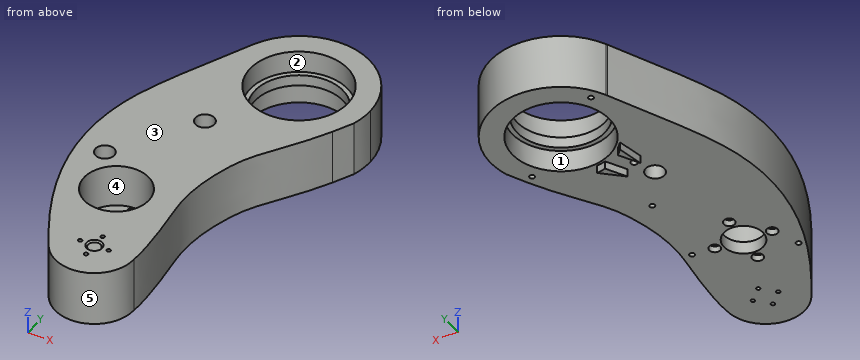
from build123d import *

# Parameters (mm, degrees)
SKIZZE1_R                        = 9
SKIZZE1_R_2                      = 28
AUFSATZ_LINEAR_AUSTRAGEN1_DEPTH  = 35
SKIZZE2_R                        = 4
SCHNITT_LINEAR_AUSTRAGEN1_DEPTH  = 1
FASE1_SIZE                       = 1
SKIZZE4_R                        = 1.25
SCHNITT_LINEAR_AUSTRAGEN2_DEPTH  = 15
SKIZZE5_R                        = 1.25
SCHNITT_LINEAR_AUSTRAGEN3_DEPTH  = 15
SKIZZE6_R                        = 12.5
SCHNITT_LINEAR_AUSTRAGEN4_DEPTH  = 35
SKIZZE7_R                        = 20.5
SCHNITT_LINEAR_AUSTRAGEN5_DEPTH  = 27
SKIZZE8_R                        = 2
SCHNITT_LINEAR_AUSTRAGEN6_DEPTH  = 15
SKIZZE9_R                        = 3.5
SCHNITT_LINEAR_AUSTRAGEN7_DEPTH  = 4
SKIZZE10_R                       = 31
SCHNITT_LINEAR_AUSTRAGEN8_DEPTH  = 14
SKIZZE11_R                       = 1.65
SCHNITT_LINEAR_AUSTRAGEN10_DEPTH = 15
SKIZZE12_R                       = 2.1
SCHNITT_LINEAR_AUSTRAGEN11_DEPTH = 15
BOSS_EXTRUDE1_DEPTH              = 5
SKETCH2_R                        = 6
CUT_EXTRUDE1_DEPTH               = 35
CUT_EXTRUDE2_START               = 8
SKETCH3_R                        = 6
CUT_EXTRUDE2_DEPTH               = 8
CUT_EXTRUDE3_START               = -10
SKETCH4_R                        = 6
CUT_EXTRUDE3_DEPTH               = 10
SKIZZE13_R                       = 1.65
SCHNITT_LINEAR_AUSTRAGEN12_DEPTH = 15


with BuildPart() as part:
    # Skizze1 → Aufsatz-Linear austragen1 (new body)
    # profile 1 of 4: a face of its own
    with BuildSketch(Plane.XY):
        with BuildLine():
            add(Edge.make_bspline(
                [(-21.90615173, -12.046597711), (-21.575742026, -12.598438537), (-21.248020936, -13.143822016), (-20.923299769, -13.682672501)],
                knots=[0.9859462, 0.9859462, 0.9859462, 0.9859462, 1, 1, 1, 1], degree=3))
            ThreePointArc((-20.923299769, -13.682672501), (7.138539969, -23.959157897), (25, 0))
            ThreePointArc((25, 0), (-6.218770247, 24.21418792), (-21.90615173, -12.046597711))
        make_face()
        Circle(SKIZZE1_R, mode=Mode.SUBTRACT)
    # profile 2 of 4: a face of its own
    with BuildSketch(Plane.XY):
        Circle(SKIZZE1_R)
    # profile 3 of 4: a face of its own
    with BuildSketch(Plane.XY):
        with BuildLine():
            ThreePointArc((-21.90615173, -12.046597711), (-6.218770247, 24.21418792), (25, 0))
            add(Edge.make_bspline(
                [(61.420827626, 153.570408345), (47.913273557, 128.743473036), (35.386108163, 117.222864261), (25.006140509, 88.46764169), (20.036125276, 66.269671918), (25.663716119, 21.50596296), (25.709290114, 4.90404347), (25, 0)],
                knots=[0.045529733, 0.045529733, 0.045529733, 0.045529733, 0.347734035, 0.409134766, 0.591243699, 0.652606584, 1, 1, 1, 1], degree=3))
            ThreePointArc((61.420827626, 153.570408345), (1.91364242, 141.373324067), (-15.526505959, 199.560222769))
            add(Edge.make_bspline(
                [(-15.526505959, 199.560222769), (-37.33502728, 155.24670183), (-72.898560815, 80.515220187), (-39.634443124, 17.562686966), (-21.90615173, -12.046597711)],
                knots=[0.001075204, 0.001075204, 0.001075204, 0.001075204, 0.231882812, 0.9859462, 0.9859462, 0.9859462, 0.9859462], degree=3))
        make_face()
    # profile 4 of 4: a face of its own
    with BuildSketch(Plane.XY):
        with BuildLine():
            ThreePointArc((-15.526505959, 199.560222769), (1.91364242, 141.373324067), (61.420827626, 153.570408345))
            add(Edge.make_bspline(
                [(67.734061127, 165.90035392), (65.561159832, 161.397385892), (63.455859297, 157.310804229), (61.420827626, 153.570408345)],
                knots=[0, 0, 0, 0, 0.045529733, 0.045529733, 0.045529733, 0.045529733], degree=3))
            ThreePointArc((67.734061127, 165.90035392), (69.429904067, 172.859718168), (70, 180))
            ThreePointArc((70, 180), (35.369713301, 223.788914648), (-15.220846491, 200.181266251))
            add(Edge.make_bspline(
                [(-15.220846491, 200.181266251), (-15.323026036, 199.973668406), (-15.424912199, 199.766654794), (-15.526505959, 199.560222769)],
                knots=[0, 0, 0, 0, 0.001075204, 0.001075204, 0.001075204, 0.001075204], degree=3))
        make_face()
        with Locations((25, 180)):
            Circle(SKIZZE1_R_2, mode=Mode.SUBTRACT)
    extrude(amount=AUFSATZ_LINEAR_AUSTRAGEN1_DEPTH)

    # Skizze2 → Schnitt-Linear austragen1 (cut)
    with BuildSketch(Plane.XY.offset(35)):
        Circle(SKIZZE2_R)
    extrude(amount=-SCHNITT_LINEAR_AUSTRAGEN1_DEPTH, mode=Mode.SUBTRACT)

    # Fase1
    fase1_edges = [part.edges().sort_by_distance(p)[0] for p in [
        (-4, 0, 35),
    ]]
    chamfer(fase1_edges, length=FASE1_SIZE - 0.0001)  # a hair under: the kernel refuses the full size

    # Skizze4 → Schnitt-Linear austragen2 (cut)
    with BuildSketch(Plane.XY.offset(35)):
        with Locations((0, 9)):
            Circle(SKIZZE4_R)
        with Locations((9, 0)):
            Circle(SKIZZE4_R)
        with Locations((0, -9)):
            Circle(SKIZZE4_R)
        with Locations((-9, 0)):
            Circle(SKIZZE4_R)
    extrude(amount=-SCHNITT_LINEAR_AUSTRAGEN2_DEPTH, mode=Mode.SUBTRACT)

    # Skizze5 → Schnitt-Linear austragen3 (cut)
    with BuildSketch(Plane(origin=(0, 0, 0), x_dir=(-1, 0, 0), z_dir=(0, 0, -1))):
        with Locations((8, 0)):
            Circle(SKIZZE5_R)
        with Locations((0, -8)):
            Circle(SKIZZE5_R)
        with Locations((-8, 0)):
            Circle(SKIZZE5_R)
        with Locations((0, 8)):
            Circle(SKIZZE5_R)
    extrude(amount=-SCHNITT_LINEAR_AUSTRAGEN3_DEPTH, mode=Mode.SUBTRACT)

    # Skizze6 → Schnitt-Linear austragen4 (cut)
    with BuildSketch(Plane.XY.offset(35)):
        with Locations((-15, 50)):
            Circle(SKIZZE6_R)
    extrude(amount=-SCHNITT_LINEAR_AUSTRAGEN4_DEPTH, mode=Mode.SUBTRACT)

    # Skizze7 → Schnitt-Linear austragen5 (cut)
    with BuildSketch(Plane.XY.offset(35)):
        with Locations((-15, 50)):
            Circle(SKIZZE7_R)
    extrude(amount=-SCHNITT_LINEAR_AUSTRAGEN5_DEPTH, mode=Mode.SUBTRACT)

    # Skizze8 → Schnitt-Linear austragen6 (cut)
    with BuildSketch(Plane.XY.offset(8)):
        with Locations((2.46462713, 51.112114754)):
            Circle(SKIZZE8_R)
        with Locations((-16.112114754, 67.46462713)):
            Circle(SKIZZE8_R)
        with Locations((-13.887885246, 32.53537287)):
            Circle(SKIZZE8_R)
        with Locations((-32.46462713, 48.887885246)):
            Circle(SKIZZE8_R)
    extrude(amount=-SCHNITT_LINEAR_AUSTRAGEN6_DEPTH, mode=Mode.SUBTRACT)

    # Skizze9 → Schnitt-Linear austragen7 (cut)
    with BuildSketch(Plane(origin=(0, 0, 0), x_dir=(-1, 0, 0), z_dir=(0, 0, -1))):
        with Locations((13.887885246, 32.53537287)):
            Circle(SKIZZE9_R)
        with Locations((-2.46462713, 51.112114754)):
            Circle(SKIZZE9_R)
        with Locations((16.112114754, 67.46462713)):
            Circle(SKIZZE9_R)
        with Locations((32.46462713, 48.887885246)):
            Circle(SKIZZE9_R)
    extrude(amount=-SCHNITT_LINEAR_AUSTRAGEN7_DEPTH, mode=Mode.SUBTRACT)

    # Skizze10 → Schnitt-Linear austragen8 (cut)
    with BuildSketch(Plane.XY.offset(35)):
        with Locations((25, 180)):
            Circle(SKIZZE10_R)
    schnitt_linear_austragen8 = extrude(amount=-SCHNITT_LINEAR_AUSTRAGEN8_DEPTH, mode=Mode.SUBTRACT)

    # Spiegeln1: Schnitt-Linear austragen8 across plane
    add(schnitt_linear_austragen8.mirror(Plane.XY.offset(17.5)), mode=Mode.SUBTRACT)

    # Skizze11 → Schnitt-Linear austragen10 (cut)
    with BuildSketch(Plane.XY):
        with Locations((12.868875195, 101.386680064)):
            Circle(SKIZZE11_R)
    extrude(amount=SCHNITT_LINEAR_AUSTRAGEN10_DEPTH, mode=Mode.SUBTRACT)

    # Skizze12 → Schnitt-Linear austragen11 (cut)
    with BuildSketch(Plane(origin=(0, 0, 0), x_dir=(-1, 0, 0), z_dir=(0, 0, -1))):
        with Locations((-2, 140)):
            Circle(SKIZZE12_R)
    extrude(amount=-SCHNITT_LINEAR_AUSTRAGEN11_DEPTH, mode=Mode.SUBTRACT)

    # Sketch1 → Boss-Extrude1 (add)
    with BuildSketch(Plane(origin=(0, 0, 0), x_dir=(-1, 0, 0), z_dir=(0, 0, -1))):
        with BuildLine():
            Line((-8.068344121, 136.51070213), (-15.214181441, 148.938245296))
            ThreePointArc((-15.214181441, 148.938245296), (-18.014496555, 148.191234041), (-20.870136061, 147.696144595))
            Line((-20.870136061, 147.696144595), (-8.068344121, 136.51070213))
        make_face()
        with BuildLine():
            ThreePointArc((0.443638721, 159.672282499), (-1.242605981, 157.724877562), (-3.077493199, 155.916841035))
            Line((-3.077493199, 155.916841035), (4.052249922, 143.517287782))
            Line((4.052249922, 143.517287782), (0.443638721, 159.672282499))
        make_face()
    extrude(amount=BOSS_EXTRUDE1_DEPTH)

    # Sketch2 → Cut-Extrude1 (cut)
    with BuildSketch(Plane(origin=(0, 0, 0), x_dir=(-1, 0, 0), z_dir=(0, 0, -1))):
        with Locations((3.710410677, 126.992836719)):
            Circle(SKETCH2_R)
    extrude(amount=-CUT_EXTRUDE1_DEPTH, mode=Mode.SUBTRACT)

    # Sketch3 → Cut-Extrude2 (cut)
    with BuildSketch(Plane(origin=(0, 0, 17.5), x_dir=(-1, 0, 0), z_dir=(0, 0, -1)).offset(CUT_EXTRUDE2_START)):
        with BuildLine():
            ThreePointArc((32.070234604, 72.232513918), (33.839840892, 80.53121825), (42.138545224, 78.761611961))
            Line((42.138545224, 78.761611961), (8.744565987, 130.257385741))
            ThreePointArc((8.744565987, 130.257385741), (9.463884926, 128.69505118), (9.710410677, 126.992836719))
            ThreePointArc((9.710410677, 126.992836719), (5.412625137, 121.23936247), (-1.323744633, 123.728287698))
            Line((-1.323744633, 123.728287698), (32.070234604, 72.232513918))
        make_face()
        with Locations((37.104389914, 75.497062939)):
            Circle(SKETCH3_R)
    extrude(amount=-CUT_EXTRUDE2_DEPTH, mode=Mode.SUBTRACT)

    # Sketch4 → Cut-Extrude3 (cut)
    with BuildSketch(Plane.XY.offset(35).offset(CUT_EXTRUDE3_START)):
        with Locations((-37.104389914, 75.497062939)):
            Circle(SKETCH4_R)
    extrude(amount=CUT_EXTRUDE3_DEPTH, mode=Mode.SUBTRACT)

    # Skizze13 → Schnitt-Linear austragen12 (cut)
    with BuildSketch(Plane(origin=(0, 0, 0), x_dir=(-1, 0, 0), z_dir=(0, 0, -1))):
        with Locations((-56.574321758, 156.900214998)):
            Circle(SKIZZE13_R)
        with Locations((6.898947223, 202.392758189)):
            Circle(SKIZZE13_R)
        with Locations((39.561746336, 32.359075962)):
            Circle(SKIZZE13_R)
        with Locations((-16.081803595, 52.359670818)):
            Circle(SKIZZE13_R)
    extrude(amount=-SCHNITT_LINEAR_AUSTRAGEN12_DEPTH, mode=Mode.SUBTRACT)


solid = part.part
Verification items for the finished model (mm, model axes). Face numbers are marked on the shaded views. A direction names the side the tool comes from. Give positions to 0.01 mm unless a question says otherwise; leave off trailing zeros.
(1) Material ranges on line 1 (Z direction, x = -21, y = 177); line 2 (Y direction, x = -10, z = 18.5); line 3 (Y direction, x = -8, z = 3.75), recorded low to high.
(2) Mould release check, pull along X, two halves, no side actions. Record for the marked faces 3, 4 and 5: +X half, -X half, draft (parallel to the pull), parting line (faces both ways), or undercut.
(3) Access from +Z, -Z, +X, -X, +Y, -Y to the whole of each face (thin tool, end or side, straight path). Record for the marked faces 1 and 2.
(4) Gauge pin test, flat ends, axial feed: pin 1 (5 mm diameter, centred on y = 167.5, z = 2.5, fed in from +X); pin 2 (4 mm diameter, centred on x = 9, y = 0, fed in from -Z); pin 3 (10 mm diameter, centred on x = -4, z = 0.5, fed in from +Y); pin 4 (3 mm diameter, centred on x = -16.11, y = 67.46, fed in from -Z). Record the tip position at first contact, or that the pin passes through.
Worked out:
1. line 1: z = 0 to 35
1. line 2: y = -22.91 to 30.12, 69.88 to 208.28
1. line 3: y = -23.69 to -1.25, 1.25 to 39.64, 60.36 to 122.8, 131.19 to 201.16, 203.62 to 210.59
2. face 3: draft
2. face 4: undercut
2. face 5: parting line
3. face 1: -Z
3. face 2: +Z
4. pin 1: stops at x = 68.87
4. pin 2: stops at z = 0
4. pin 3: stops at y = 218.07
4. pin 4: passes through
